Build history of the part. All positions in model axes, mm. Give positions to 0.01 mm unless a question says otherwise; leave off trailing zeros. Order: outer loops, then holes, each group sorted by start corner. A loop starts at its lowest first (then second) coordinate and runs counter-clockwise, first axis right, second up. Notation, with made-up numbers: M 51,47.25 L 86,47.25 A22 ccw 86,81.25 Z; hole C -35,0 d3. An arc over 180 degrees is marked long. One line per item, written item: value.
Autodesk Inventor part; units mm, degrees
ref_plane "YZ Plane" through (0, 0, 0) normal (1, 0, 0) x (0, 1, 0)
ref_plane "XZ Plane" through (0, 0, 0) normal (0, 1, 0) x (-1, 0, 0)
ref_plane "XY Plane" through (0, 0, 0) normal (0, 0, 1) x (1, 0, 0)
sketch "Sketch1" plane through (0, 0, 0) normal (0, 1, 0) x (-1, 0, 0)
  line L0 (6.35, -3.6662) -> (0, -7.3323)
  line L1 (0, -7.3323) -> (-6.35, -3.6662)
  line L2 (-6.35, -3.6662) -> (-6.35, 3.6662)
  line L3 (-6.35, 3.6662) -> (0, 7.3323)
  line L4 (0, 7.3323) -> (6.35, 3.6662)
  line L5 (6.35, 3.6662) -> (6.35, -3.6662)
  point P0 (0, 0)
  point P1 (0, 0)
  point P2 (0, 0)
  dimension "d0" = 12.7
extrude "Extrusion1" add sketch "Sketch1" along normal blind 567.309
sketch "Sketch2" plane through (0, 0, 0) normal (0, -1, 0) x (1, 0, 0)
  point P0 (0, 0)
  point P1 (0, 0)
hole "Hole1" at (0, 0, 0) direction (0, 1, 0) diameter 4.9784 depth 25.4
sketch "Sketch3" plane through (0, 567.309, 0) normal (0, 1, 0) x (1, 0, 0)
  point P0 (0, 0)
  point P1 (0, 0)
hole "Hole2" at (0, 567.309, 0) direction (0, -1, 0) diameter 4.9784 depth 25.4
properties part number "INTK_004_HexShaft6" material "Aluminum 6061"
1) Saw through at A-A, the plane z = 0. Write the cut outline in (x, y), then the cut area to 3 significant figures.
Check values:
outline: M -6.35,0 L -2.49,0 L -2.49,25.4 L 2.49,25.4 L 2.49,0 L 6.35,0 L 6.35,567.31 L 2.49,567.31 L 2.49,541.91 L -2.49,541.91 L -2.49,567.31 L -6.35,567.31 Z
area: 6,950 mm^2
2) Pin check, flat tips, straight feed: pin 1 (2 mm diameter, centred on x = 3, z = -4.5, fed in from -Y); pin 2 (1 mm diameter, centred on x = 2, y = 266.5, fed in from +Z); pin 3 (4 mm diameter, centred on x = -0.5, y = 296, fed in from -Z); pin 4 (6 mm diameter, centred on x = 5, y = 93, fed in from -Z). Stop position of each tip, or through.
Check values:
pin 1: y = 0
pin 2: z = 6.47
pin 3: z = -7.33
pin 4: z = -6.18
3) Saw through at B-B, the plane y = 314. Write the cut outline in (x, z), then the cut area to 3 significant figures.
Check values:
outline: M -6.35,-3.67 L 0,-7.33 L 6.35,-3.67 L 6.35,3.67 L 0,7.33 L -6.35,3.67 Z
area: 140 mm^2
4) Drill centre lines: probe 1 along Z at (x, y) = (0, 551.5); probe 2 along X at (y, z) = (10.5, 0); probe 3 along Y at (x, z) = (0.5, 2). Where is each one in solid material? Low to high. Write a range as from..to.
Check values:
probe 1: -7.33..-2.49, 2.49..7.33
probe 2: -6.35..-2.49, 2.49..6.35
probe 3: 25.4..541.91
